Verification items for the finished model (mm, model axes). A direction names the side the tool comes from. Coordinates: 2 decimals unless noted, no trailing zeros. Order: outer loops, then holes, each group sorted by start corner. A loop starts at its lowest first (then second) coordinate and runs counter-clockwise, first axis right, second up.
Q1. Draft check along X on faces 3 (the cylindrical face through (0.186, 0.76, -6.587)), 4 (the cylindrical face through (-1.08, 6.18, -4.88)), 5 (the flat face through (0, 11.5, 4)). Enter one of: pulls with the +X half, pulls with the -X half, needs draft (parallel to the pull), parting line crosses it, or undercut.
Q2. Cross-section at C-C, the plane x = 7. Record the boundary of the cut face in (y, z).
Q3. Depth check by flat-ended pin: P1, Ø6, axis at x = 7.5, z = -2, coming from the -Y side; P2, Ø6, axis at y = 5, z = 4.5, coming from the -X side; P3, Ø2.5, axis at x = -8, z = 0, coming from the -Y side; P4, Ø3, axis at y = 2, z = -8, coming from the +X side. Enter the tip coordinate at first touch or a pass-through.
Q4. Cross-section at A-A, the plane x = 0. Record the boundary of the cut face in (y, z) (3 decimals).
Q5. Thickness scan on line 1 (Y direction, x = 4.5, z = -5.5); line 2 (X direction, y = 0.85, z = 8) (3 decimals). Record the ranges inside material, lowest first.
Q6. Cross-section at D-D, the plane y = 9. Record the boundary of the cut face in (x, z), and give its area (3 significant figures).
Q7. Cross-section at B-B, the plane z = 0. Record the boundary of the cut face in (x, y) (3 decimals), and give its area (3 significant figures).
Q8. Set-up check for faces 1 (the cylindrical face through (-0.186, 0.76, 6.587)), 2 (the flat face through (-2, 1.5, -5)): record each of +Z, -Z, +X, -X, +Y, -Y from which the full face is reachable in a straight line by a thin tool's end or side.
Autodesk Inventor part; units mm, degrees
ref_plane "YZ Plane" through (0, 0, 0) normal (1, 0, 0) x (0, 1, 0)
ref_plane "XZ Plane" through (0, 0, 0) normal (0, 1, 0) x (-1, 0, 0)
ref_plane "XY Plane" through (0, 0, 0) normal (0, 0, 1) x (1, 0, 0)
sketch "Sketch1" plane through (0, 0, 0) normal (0, 1, 0) x (-1, 0, 0)
  circle A0 centre (0, 0) radius 11
  dimension "d0" = 22
extrude "Extrusion1" add sketch "Sketch1" along normal blind 1.5
sketch "Sketch2" plane through (0, 1.5, 0) normal (0, 1, 0) x (1, 0, 0)
  circle A0 centre (0, 0) radius 5
  circle A1 centre (0, 0) radius 3
  dimension "d3" = 10
  dimension "d4" = 6
extrude "Extrusion2" add sketch "Sketch2" along normal blind 10
sketch "Sketch3" plane through (0, 1.5, 0) normal (0, 1, 0) x (1, 0, 0)
  circle A0 centre (0, 0) radius 3
  dimension "d7" = 6
extrude "Extrusion3" cut sketch "Sketch3" against normal blind 1.5
sketch "Sketch4" plane through (0, 1.5, 0) normal (0, 1, 0) x (1, 0, 0)
  circle A0 centre (0, -8) radius 1.425
  line L0 (0, 0) -> (0, -8)
  line L1 (0, 0) -> (-11, 0)
  circle A1 centre (0, 0) radius 11
  dimension "d10" = 2.85
  dimension "d11" = 8
extrude "Extrusion4" cut sketch "Sketch4" against normal blind 1.5 contours A0
pattern_circular "Circular Pattern1" count 4 over 360 about axis through (0, 1.5, 0) along (0, 1, 0) of "Extrusion4"
fillet "Fillet1" radius 0.5 1 edges at (-3, 11.5, 0)
fillet "Fillet2" radius 0.5 1 edges at (-5, 11.5, 0)
properties part number "Stepper_Coupler"
Check values:
1. face 3: undercut
1. face 4: parting line crosses it
1. face 5: needs draft
2. outline: (0, -8.49) - (1.5, -8.49) - (1.5, -1.02) - (0, -1.02) - close; (0, 1.02) - (1.5, 1.02) - (1.5, 8.49) - (0, 8.49) - close
3. P1: stops at y = 0
3. P2: stops at x = -4.77
3. P3: passes through
3. P4: stops at x = 8.81
4. outline: (0, -11) - (1.5, -11) - (1.5, -9.425) - (0, -9.425) - close; (0, -6.575) - (1.5, -6.575) - (1.5, -5) - (11, -5) arc R0.5 ccw to (11.5, -4.5) - (11.5, -3.5) arc R0.5 ccw to (11, -3) - (0, -3) - close; (0, 3) - (11, 3) arc R0.5 ccw to (11.5, 3.5) - (11.5, 4.5) arc R0.5 ccw to (11, 5) - (1.5, 5) - (1.5, 6.575) - (0, 6.575) - close; (0, 9.425) - (1.5, 9.425) - (1.5, 11) - (0, 11) - close
5. line 1: y = 0 to 1.5
5. line 2: x = -7.55 to -1.425, 1.425 to 7.55
6. outline: circle Ø10 at (0, 0); hole circle Ø6 at (0, 0)
6. area: 50.3 mm2
7. outline: (-11, 0) - (-9.425, 0) - (-9.425, 1.5) - (-11, 1.5) - close; (-6.575, 0) - (-3, 0) - (-3, 11) arc R0.5 ccw to (-3.5, 11.5) - (-4.5, 11.5) arc R0.5 ccw to (-5, 11) - (-5, 1.5) - (-6.575, 1.5) - close; (3, 0) - (6.575, 0) - (6.575, 1.5) - (5, 1.5) - (5, 11) arc R0.5 ccw to (4.5, 11.5) - (3.5, 11.5) arc R0.5 ccw to (3, 11) - close; (9.425, 0) - (11, 0) - (11, 1.5) - (9.425, 1.5) - close
7. area: 55.2 mm2
8. face 1: +Y, -Y
8. face 2: +Y
